The drawing under review shows one solid part. Ordinate dimensions are in mm from its lowest x, y, z. Round coordinates to 2 decimals unless told otherwise and drop trailing zeros. Loops run counter-clockwise (first coordinate to the right, second up) from the corner with the lowest first, then second, coordinate; pieces in that order, holes last. Notation, with made-up numbers: (43, 22.5) -> (83, 22.5) arc R17 ccw to (83, 49.5) -> close; hole circle Ø1 at (-40, -21). An arc over 180 degrees is marked (long way). Answer as CSV lines item,"result". Start each with the question number.
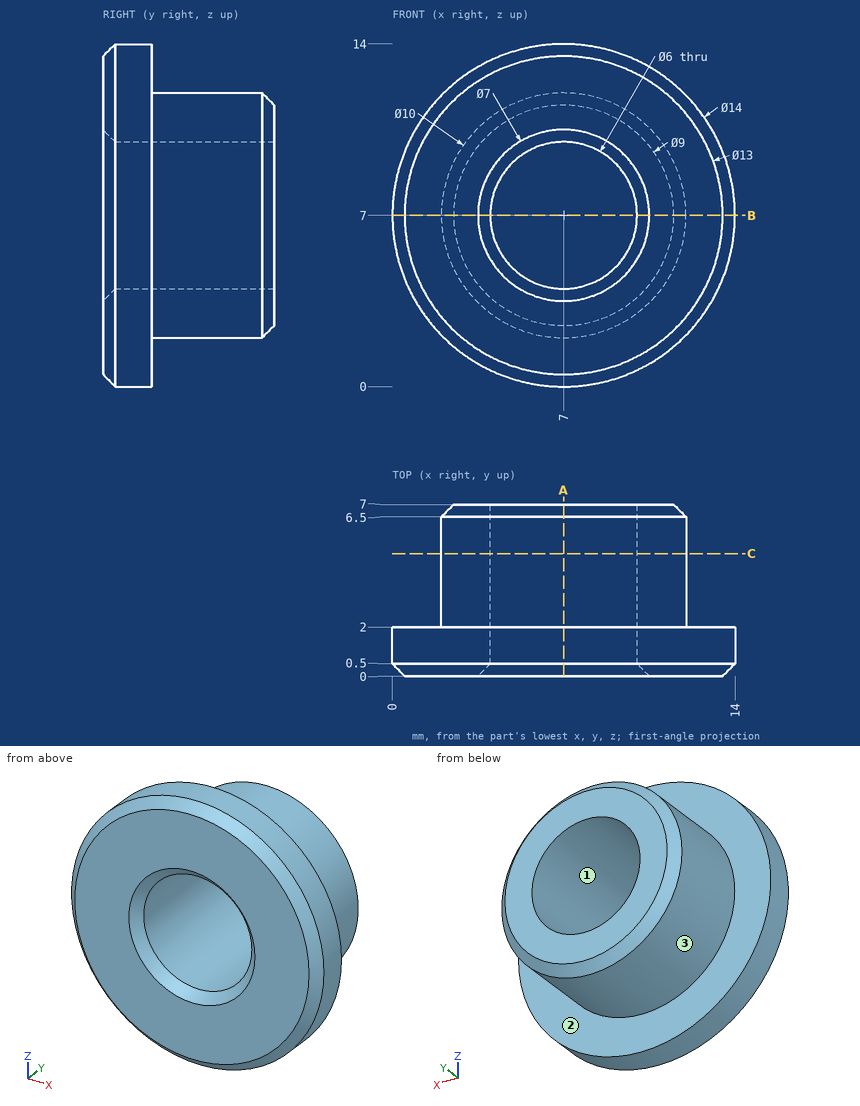
Q1. Add section B-B, the plane z = 7. Give the boundary of the cut face in (x, y).
Q2. To check wall thickness, follow probe 1 along Z at (x, y) = (7, 3.25); probe 2 along Y at (x, z) = (1.25, 4.25). State the ranges of each line that lie inside material, in increasing order. Write a range as from..to.
Q3. Mouldability with a two-part tool opening along Z and no side actions: class the marked faces 1, 2 and 3 as pulls with the +Z half, pulls with the -Z half, needs draft (parallel to the pull), parting line crosses it, or undercut.
Q4. Add section C-C, the plane y = 5. Give the boundary of the cut face in (x, z), and give its area (3 significant figures).
Q5. Add section A-A, the plane x = 7. Give the boundary of the cut face in (y, z).
Worked answers:
1,outline,"(0, 0.5) -> (0.5, 0) -> (3.5, 0) -> (4, 0.5) -> (4, 7) -> (2.5, 7) -> (2, 6.5) -> (2, 2) -> (0, 2) -> close; (10, 0.5) -> (10.5, 0) -> (13.5, 0) -> (14, 0.5) -> (14, 2) -> (12, 2) -> (12, 6.5) -> (11.5, 7) -> (10, 7) -> close"
2,probe 1,"z = 2..4, 10..12"
2,probe 2,"y = 0..2"
3,face 1,"undercut"
3,face 2,"needs draft"
3,face 3,"parting line crosses it"
4,outline,"circle Ø10 at (7, 7); hole circle Ø6 at (7, 7)"
4,area,"50.3 mm^2"
5,outline,"(0, 0.5) -> (0.5, 0) -> (2, 0) -> (2, 2) -> (6.5, 2) -> (7, 2.5) -> (7, 4) -> (0.5, 4) -> (0, 3.5) -> close; (0, 10.5) -> (0.5, 10) -> (7, 10) -> (7, 11.5) -> (6.5, 12) -> (2, 12) -> (2, 14) -> (0.5, 14) -> (0, 13.5) -> close"
